Geometry check sheet. Reference: the model listing, model coordinates, mm. A direction names the side the tool comes from. Coordinates: 2 decimals unless noted, no trailing zeros. Order: outer loops, then holes, each group sorted by start corner. A loop starts at its lowest first (then second) coordinate and runs counter-clockwise, first axis right, second up. Notation, with made-up numbers: M 56,70.25 L 69,70.25 A16 cw 69,93.25 Z; hole C 43,-37 d5. An arc over 180 degrees is marked long. One line per item, written item: value. Start each with the question number.
1) Thickness scan on L1, parallel to Z at x = -12.7, y = -1.75 (3 decimals); L2, parallel to Z at x = 41, y = 1 (3 decimals); L3, parallel to X at y = 1, z = 4. Record the ranges inside material, lowest first. Write a range as from..to.
2) Sectioned sample at D-D, the plane x = 48. Enter the section's corners in (y, z) (3 decimals).
3) Access from +Z, -Z, +X, -X, +Y, -Y to the whole of each face (thin tool, end or side, straight path). Record for faces 5 (the flat face through (38, 0, -9.525)), 6 (the flat face through (-1, 3.175, 0)).
4) Draft check along Z on faces 1 (the cylindrical face through (-61.5, 0.81, 8.44)), 2 (the flat face through (-1, 0, -15.875)), 3 (the cylindrical face through (58.727, 0.809, -9.595)), 4 (the flat face through (-1, -3.175, 0)). Enter one of: pulls with the +Z half, pulls with the -Z half, needs draft (parallel to the pull), parting line crosses it, or undercut.
5) Sectioned sample at A-A, the plane z = 0. Enter the section's corners in (x, y) (3 decimals).
6) Go/stop test with flat-tipped pins: P1, Ø3, axis at x = -12.7, z = 9.525, coming from the +Y side (3 decimals); P2, Ø3, axis at x = 60.325, z = -9.525, coming from the +Y side; P3, Ø5, axis at x = -60.325, z = 9.525, coming from the -Y side (3 decimals). Record where each tip stops, or that it passes through.
7) Sectioned sample at C-C, the plane x = -12.7. Enter the section's corners in (y, z) (3 decimals), then the cut area to 3 significant figures.
8) Sectioned sample at B-B, the plane y = 2. State how many separate pieces and enclosed holes the cut face has, then the cut area to 3 significant figures.
```python
from build123d import *

# Parameters (mm, degrees)
SKETCH1_W                                       = 127
SKETCH1_H                                       = 31.75
BOSS_EXTRUDE1_DEPTH                             = 3.175
CSK_FOR_M3_FLAT_HEAD_MACHINE_SCREW1_D           = 3.2
CSK_FOR_M3_FLAT_HEAD_MACHINE_SCREW1_DEPTH       = 12.7
CSK_FOR_M3_FLAT_HEAD_MACHINE_SCREW1_CSINK_D     = 6.3
CSK_FOR_M3_FLAT_HEAD_MACHINE_SCREW1_CSINK_ANGLE = 90
CSK_FOR_M3_FLAT_HEAD_MACHINE_SCREW1_TIP         = 0.96137699
M3X0_5_TAPPED_HOLE1_D                           = 2.5
CUT_EXTRUDE1_DEPTH                              = 66.761600688


with BuildPart() as part:
    # Sketch1 → Boss-Extrude1 (new, symmetric)
    with BuildSketch(Plane(origin=(0, 0, 0), x_dir=(1, 0, 0), z_dir=(0, 1, 0))):
        Rectangle(SKETCH1_W, SKETCH1_H)
    extrude(amount=BOSS_EXTRUDE1_DEPTH, both=True)

    # CSK for M3 Flat Head Machine Screw1
    with Locations(Plane(origin=(0, -3.175, 0), x_dir=(-1, 0, 0), z_dir=(0, -1, 0))):
        with Locations((60.325, 9.525), (60.325, -9.525), (-60.325, -9.525), (-60.325, 9.525)):
            CounterSinkHole(CSK_FOR_M3_FLAT_HEAD_MACHINE_SCREW1_D / 2, CSK_FOR_M3_FLAT_HEAD_MACHINE_SCREW1_CSINK_D / 2, depth=CSK_FOR_M3_FLAT_HEAD_MACHINE_SCREW1_DEPTH, counter_sink_angle=CSK_FOR_M3_FLAT_HEAD_MACHINE_SCREW1_CSINK_ANGLE)
            with Locations((0, 0, -(CSK_FOR_M3_FLAT_HEAD_MACHINE_SCREW1_DEPTH + CSK_FOR_M3_FLAT_HEAD_MACHINE_SCREW1_TIP / 2))):  # 118° drill point
                Cone(0, CSK_FOR_M3_FLAT_HEAD_MACHINE_SCREW1_D / 2, CSK_FOR_M3_FLAT_HEAD_MACHINE_SCREW1_TIP, mode=Mode.SUBTRACT)

    # M3x0.5 Tapped Hole1 (through all)
    with Locations(Plane(origin=(0, 3.175, 0), x_dir=(1, 0, 0), z_dir=(0, 1, 0))):
        with Locations((-12.7, 9.525), (12.7, 9.525), (12.7, -9.525), (-12.7, -9.525)):
            Hole(M3X0_5_TAPPED_HOLE1_D / 2)

    # Sketch10 → Cut-Extrude1 (cut, through all)
    with BuildSketch(Plane(origin=(0, 3.175, 0), x_dir=(1, 0, 0), z_dir=(0, 1, 0))):
        with BuildLine():
            Line((-44.45, 9.525), (-31.75, 9.525))
            ThreePointArc((-31.75, 9.525), (-22.225, 0), (-31.75, -9.525))
            Line((-31.75, -9.525), (-44.45, -9.525))
            ThreePointArc((-44.45, -9.525), (-53.975, 0), (-44.45, 9.525))
        make_face()
        with BuildLine():
            Line((44.45, -9.525), (31.75, -9.525))
            ThreePointArc((31.75, -9.525), (22.225, 0), (31.75, 9.525))
            Line((31.75, 9.525), (44.45, 9.525))
            ThreePointArc((44.45, 9.525), (53.975, 0), (44.45, -9.525))
        make_face()
    extrude(amount=-CUT_EXTRUDE1_DEPTH, mode=Mode.SUBTRACT)


solid = part.part
```
Final values:
1. L1: z = -15.875..-10.775, -8.275..8.275, 10.775..15.875
1. L2: z = -15.875..-9.525, 9.525..15.875
1. L3: x = -63.5..-53.09, -23.11..23.11, 53.09..63.5
2. outline: M -3.175,-15.875 L 3.175,-15.875 L 3.175,-8.839 L -3.175,-8.839 Z; M -3.175,8.839 L 3.175,8.839 L 3.175,15.875 L -3.175,15.875 Z
3. face 5: +Y, -Y
3. face 6: +Z, -Z, +X, -X, +Y
4. face 1: undercut
4. face 2: pulls with the -Z half
4. face 3: undercut
4. face 4: needs draft
5. outline: M -63.5,-3.175 L -53.975,-3.175 L -53.975,3.175 L -63.5,3.175 Z; M -22.225,-3.175 L 22.225,-3.175 L 22.225,3.175 L -22.225,3.175 Z; M 53.975,-3.175 L 63.5,-3.175 L 63.5,3.175 L 53.975,3.175 Z
6. P1: stops at y = 3.175
6. P2: passes through
6. P3: stops at y = -2.525
7. outline: M -3.175,-15.875 L 3.175,-15.875 L 3.175,-10.775 L -3.175,-10.775 Z; M -3.175,-8.275 L 3.175,-8.275 L 3.175,8.275 L -3.175,8.275 Z; M -3.175,10.775 L 3.175,10.775 L 3.175,15.875 L -3.175,15.875 Z
7. area: 170 mm^2
8. separate pieces: 1
8. enclosed holes: 10
8. area: 2,930 mm^2
